Job drawing, mm, ordinate dimensions from the low corner. One solid piece. Round coordinates to 2 decimals unless told otherwise and drop trailing zeros. Write each loop counter-clockwise with the first axis right and the second up, starting at its lowest first coordinate (ties: lowest second). Pieces come first, ordered by that corner, then holes.
1) Drill centre lines: L1, parallel to Y at x = 19, z = 8; L2, parallel to Y at x = 76.5, z = 3; L3, parallel to X at y = 16, z = 26.5. Where is each one in solid material? Low to high.
2) Saw through at A-A on z = 5.5. Write the cut outline in (x, y).
3) Flat gauge pin, fed straight in: pin 1 (1.5 mm diameter, centred on x = 15, z = 14, fed in from +Y). Where does the tip first touch, or does it go through?
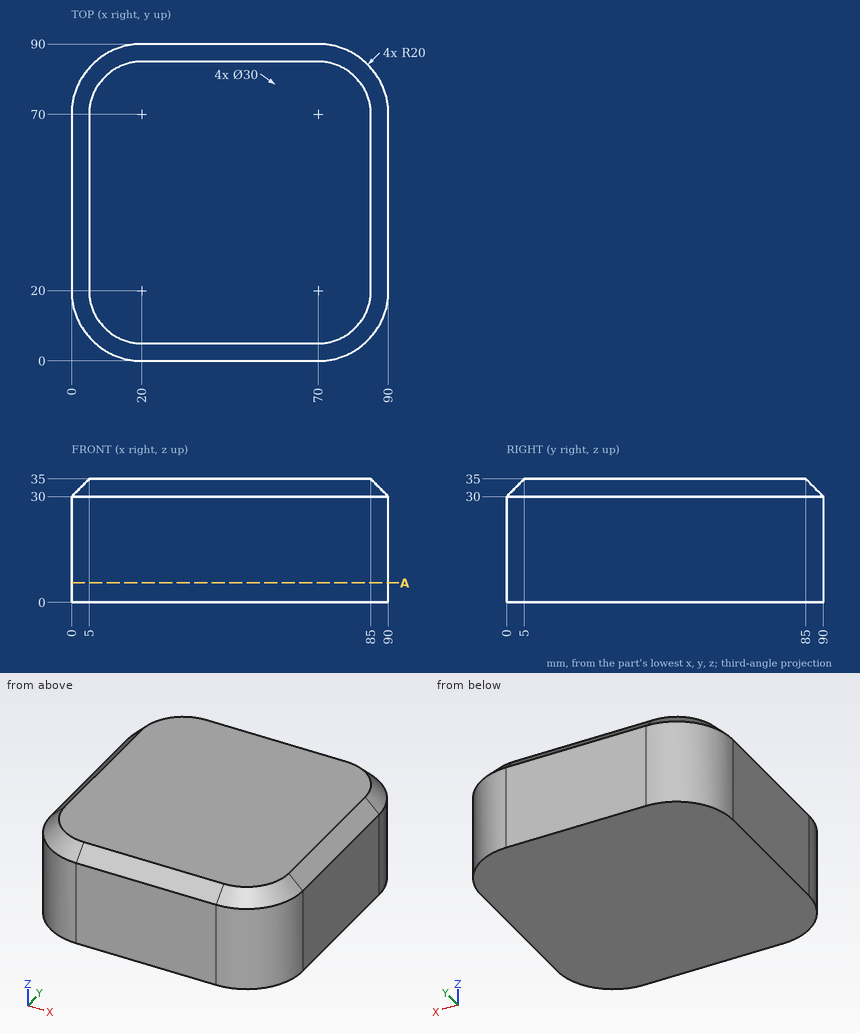
Completed:
1. L1: y = 0.03 to 89.97
1. L2: y = 1.09 to 88.91
1. L3: x = 0.4 to 89.6
2. outline: (0, 20) arc R20 ccw to (20, 0) - (70, 0) arc R20 ccw to (90, 20) - (90, 70) arc R20 ccw to (70, 90) - (20, 90) arc R20 ccw to (0, 70) - close
3. pin 1: stops at y = 89.54
